from build123d import *

# Parameters (mm, degrees)
F0_R     = 7
F1_DEPTH = 8
F2_R     = 7.75
F2_R_2   = 7
F3_DEPTH = 1
F4_R     = 7.75
F4_R_2   = 7
F5_DEPTH = 1
F6_R     = 0.99999


# Not quite as in the source:
# - a fillet or chamfer is up to 0.001 mm smaller than in the source, because OpenCascade refuses the exact size


with BuildPart() as f1:
    # F0 (on Front) → F1 (new body, symmetric)
    with BuildSketch(Plane.XZ):
        Circle(F0_R)
    extrude(amount=F1_DEPTH, both=True)

    # F2 (on face) → F3 (join)
    with BuildSketch(Plane.XZ.offset(8)):
        Circle(F2_R)
        Circle(F2_R_2, mode=Mode.SUBTRACT)
        Circle(F2_R_2)
    extrude(amount=F3_DEPTH)

    # F4 (on face) → F5 (join)
    with BuildSketch(Plane(origin=(0, 8, 0), x_dir=(-1, 0, 0), z_dir=(0, 1, 0))):
        Circle(F4_R)
        Circle(F4_R_2, mode=Mode.SUBTRACT)
        Circle(F4_R_2)
    extrude(amount=F5_DEPTH)

    # F6 (radius 1 in the source; OpenCascade refuses exactly that, so slightly less here)
    f6_edges = [f1.edges().sort_by_distance(p)[0] for p in [
        (-7.75, -9, 0),
        (7.75, 9, 0),
    ]]
    fillet(f6_edges, radius=F6_R)


solid = f1.part
The listing builds one solid part. Answer for the finished solid, in the listing's coordinates (mm). Give positions to 0.01 mm unless a question says otherwise; leave off trailing zeros. Order: outer loops, then holes, each group sorted by start corner. A loop starts at its lowest first (then second) coordinate and runs counter-clockwise, first axis right, second up. Notation, with made-up numbers: (-10.5, -17) - (42.5, -17) arc R22 ccw to (42.5, 7) - close; hole circle Ø6 at (56.25, 19). An arc over 180 degrees is marked (long way). One line per item, written item: value. Start each with the question number.
1) Given pin 1 Ø4 at (y, z) = (1.5, 3) entering from -X; pin 2 Ø2 at (x, y) = (0.5, 2.5) entering from -Z; pin 3 Ø6 at (x, y) = (-4, 0) entering from +Z, each flat-ended and moving along its own axis, determine where each tip first touches the part or whether it passes through.
2) The mould has two halves that part along Y. Classify faces 1 (the face through (0, -9, 0)), 2 (the face through (0, 9, 0)), 3 (the face through (6, 8, -4)): released by +Y, released by -Y, zero draft, split by the parting line, or undercut.
3) Find the intervals of material crossed by L1, parallel to Y at x = -3.25, z = -6; L2, parallel to X at y = -1, z = -0.25; L3, parallel to Y at x = 4.75, z = -6, in increasing order.
4) A cutting plane is placed at C-C on y = 7.5. Give the vertices of the cut face in (x, z), then the cut area to 3 significant figures.
Answer sheet:
1. pin 1: stops at x = -6.93
1. pin 2: stops at z = -7
1. pin 3: stops at z = 6.93
2. face 1: released by -Y
2. face 2: released by +Y
2. face 3: undercut
3. L1: y = -9 to 9
3. L2: x = -7 to 7
3. L3: y = -8.43 to -8, 8 to 8.43
4. outline: circle Ø14 at (0, 0)
4. area: 154 mm2
